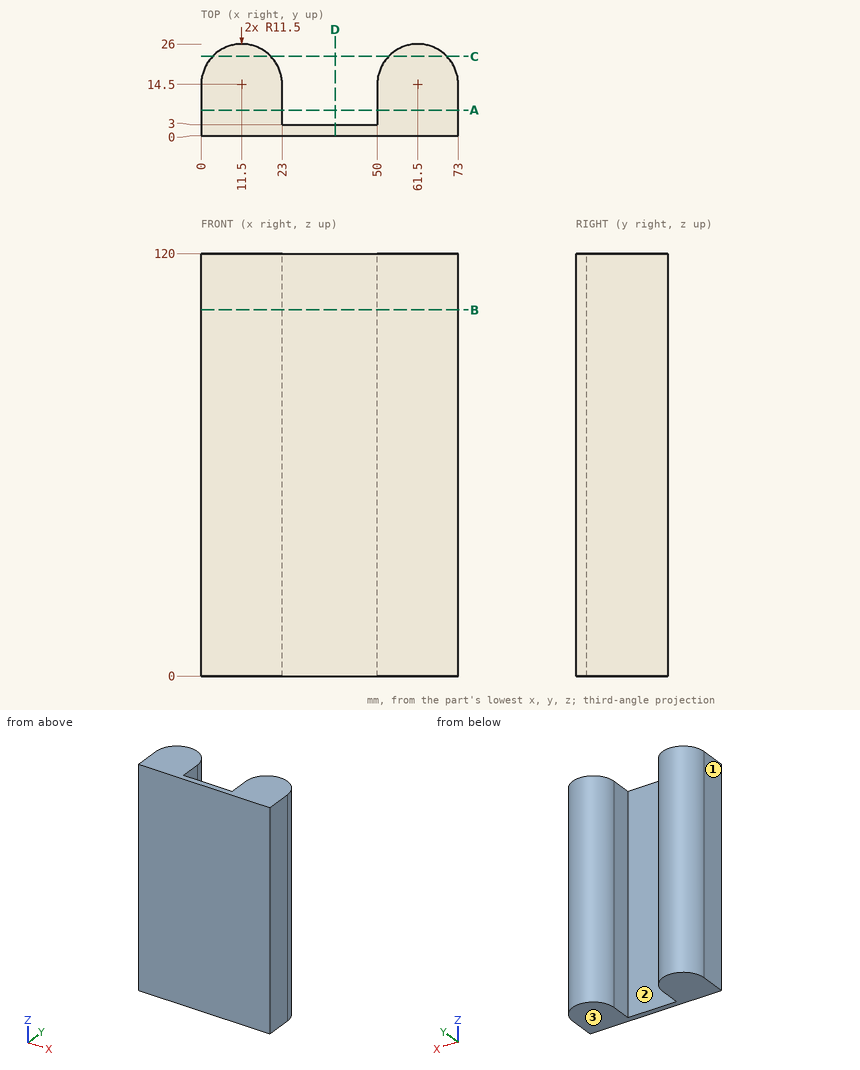
Drawing for the job (mm, zero at the part's lowest x, y, z). Give positions to 0.01 mm unless a question says otherwise; leave off trailing zeros. Loops run counter-clockwise (first coordinate to the right, second up) from the corner with the lowest first, then second, coordinate; pieces in that order, holes last. Notation, with made-up numbers: (-14.5, 72.5) - (-8.5, 72.5) arc R17 ccw to (-8.5, 85.5) - close; hole circle Ø6 at (43.25, 89). An arc over 180 degrees is marked (long way). Write item = value, one per line. Start each with the question number.
1) Band-saw the part on C-C on y = 22.5. Give the cut face in (x, z), plus the area to 3 significant figures.
2) Pull direction X, two halves, no side cores. Call the marked faces 1, 2 and 3: +X half, -X half, draft (parallel to the pull), parting line (faces both ways), or undercut.
3) Drop flat-ended pins along their axis: pin 1 Ø4 at (x, z) = (31, 106.5) entering from +Y; pin 2 Ø1.5 at (x, z) = (62.5, 29.5) entering from +Y; pin 3 Ø21.5 at (x, z) = (43, 81) entering from +Y. Give the stop position or say it passes through.
4) Band-saw the part on A-A on y = 7.25. Give the cut face in (x, z), plus the area to 3 significant figures.
5) Band-saw the part on D-D on x = 38. Give the cut face in (y, z).
6) Probe probe 1 along X at (y, z) = (9.25, 66); probe 2 along X at (y, z) = (17, 79); probe 3 along Y at (x, z) = (40, 111). List the from-to ranges inside material, lowest first. Write a range as from..to.
7) Band-saw the part on B-B on z = 104. Give the cut face in (x, y), plus the area to 3 significant figures.
Final values:
q1.outline = (3.24, 0) - (19.76, 0) - (19.76, 120) - (3.24, 120) - close; (53.24, 0) - (69.76, 0) - (69.76, 120) - (53.24, 120) - close
q1.area = 3,970 mm²
q2.face_1 = -X half
q2.face_2 = undercut
q2.face_3 = draft
q3.pin_1 = 3
q3.pin_2 = 26
q3.pin_3 = 23
q4.outline = (0, 0) - (23, 0) - (23, 120) - (0, 120) - close; (50, 0) - (73, 0) - (73, 120) - (50, 120) - close
q4.area = 5,520 mm²
q5.outline = (0, 0) - (3, 0) - (3, 120) - (0, 120) - close
q6.probe_1 = 0..23, 50..73
q6.probe_2 = 0.28..22.72, 50.28..72.72
q6.probe_3 = 0..3
q7.outline = (0, 0) - (73, 0) - (73, 14.5) arc R11.5 ccw to (50, 14.5) - (50, 3) - (23, 3) - (23, 14.5) arc R11.5 ccw to (0, 14.5) - close
q7.area = 1,160 mm²
